Part model, mm, in its own coordinate system. Round coordinates to 2 decimals unless told otherwise and drop trailing zeros. Write each loop counter-clockwise with the first axis right and the second up, starting at its lowest first coordinate (ties: lowest second). Pieces come first, ordered by that corner, then holes. Notation, with made-up numbers: (82, -28) -> (91, -28) arc R16 ccw to (91, 2) -> close; hole circle Ø4 at (-9, 21). An arc over 180 degrees is marked (long way). Return JSON: item names as keys, results as strings. Group by question number.
(1) Drill centre lines: L1, parallel to Y at x = 18, z = 0.3; L2, parallel to Y at x = 15.25, z = 0.7; L3, parallel to X at y = -15, z = 1.25. Where is each one in solid material? Low to high. Write a range as from..to.
(2) Saw through at A-A (y = -15.25). List the corners of the cut face in (x, z), plus the area to 3 significant figures.
(3) Saw through at D-D (x = 5). List the corners of the cut face in (y, z).
(4) Saw through at B-B (x = -11). List the corners of the cut face in (y, z).
(5) Saw through at C-C (z = 0.8). State how many separate pieces and enclosed holes the cut face has, plus the area to 3 significant figures.
from build123d import *

# Parameters (mm, degrees)
F0_R     = 1.5
F0_R_2   = 3.25
F1_DEPTH = 1.5


# Not quite as in the source:
# - ends of sketch curves that miss each other by under 0.0002 mm in the source are joined


with BuildPart() as f1:
    # F0 (on Top) → F1 (new body)
    with BuildSketch(Plane.XY):
        with BuildLine():
            ThreePointArc((6.3250610024, 28.8463679906), (-4.837e-07, 28.033009), (-6.3250619384, 28.8463682354))
            Line((-6.3250619384, 28.8463682354), (-16.589434, 31.530609))
            ThreePointArc((-16.589434, 31.530609), (-20.910174001, 30.6508727545), (-22.854447, 26.693281))
            Line((-22.854447, 26.693281), (-22.854447, -26.693281))
            ThreePointArc((-22.854447, -26.693281), (-20.910174001, -30.6508727545), (-16.5894340018, -31.5306089933))
            Line((-16.5894340018, -31.5306089933), (-6.325062, -28.846368))
            ThreePointArc((-6.325062, -28.846368), (-4.837e-07, -28.033009), (6.3250610024, -28.8463679906))
            Line((6.3250610024, -28.8463679906), (16.589434, -31.530609))
            ThreePointArc((16.589434, -31.530609), (20.9101733838, -30.6508724589), (22.854446, -26.693281))
            Line((22.854446, -26.693281), (22.854446, 26.693281))
            ThreePointArc((22.854446, 26.693281), (20.9101733838, 30.6508724589), (16.5894339378, 31.530609238))
            Line((16.5894339378, 31.530609238), (6.3250610024, 28.8463679906))
        make_face()
        with Locations((-17.854447, -26.693281)):
            Circle(F0_R, mode=Mode.SUBTRACT)
        with Locations((-15.25, -15.25)):
            Circle(F0_R, mode=Mode.SUBTRACT)
        with Locations((-11, -3.5)):
            Circle(F0_R, mode=Mode.SUBTRACT)
        with Locations((5, -23.033009)):
            Circle(F0_R_2, mode=Mode.SUBTRACT)
        with Locations((17.854446, -26.693281)):
            Circle(F0_R, mode=Mode.SUBTRACT)
        with Locations((11, -3.5)):
            Circle(F0_R, mode=Mode.SUBTRACT)
        with Locations((15.25, -15.25)):
            Circle(F0_R, mode=Mode.SUBTRACT)
        with Locations((-15.25, 15.25)):
            Circle(F0_R, mode=Mode.SUBTRACT)
        with Locations((-11, 11.5)):
            Circle(F0_R, mode=Mode.SUBTRACT)
        with Locations((-17.854447, 26.693281)):
            Circle(F0_R, mode=Mode.SUBTRACT)
        with Locations((11, 11.5)):
            Circle(F0_R, mode=Mode.SUBTRACT)
        with Locations((15.25, 15.25)):
            Circle(F0_R, mode=Mode.SUBTRACT)
        with Locations((17.854446, 26.693281)):
            Circle(F0_R, mode=Mode.SUBTRACT)
    extrude(amount=F1_DEPTH)


solid = f1.part
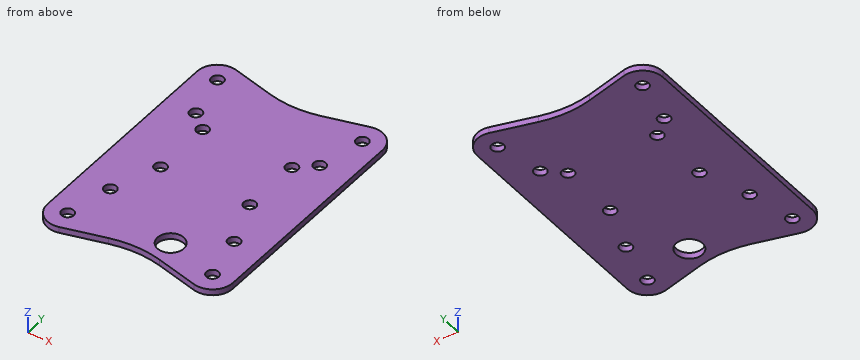
Computed values:
{
 "1": {"L1": "-31.69..-28.19, -25.2..25.2, 28.19..31.69", "L2": "-31.18..-16.75, -13.75..13.75, 16.75..31.18", "L3": "-22.85..-16.73, -13.77..13.77, 16.73..22.85"},
 "2": {"outline": "(-22.85, 0) -> (-16.75, 0) -> (-16.75, 1.5) -> (-22.85, 1.5) -> close; (-13.75, 0) -> (13.75, 0) -> (13.75, 1.5) -> (-13.75, 1.5) -> close; (16.75, 0) -> (22.85, 0) -> (22.85, 1.5) -> (16.75, 1.5) -> close", "area": "59.6 mm2"},
 "3": {"outline": "(-28.54, 0) -> (-26.28, 0) -> (-26.28, 1.5) -> (-28.54, 1.5) -> close; (-19.78, 0) -> (28.54, 0) -> (28.54, 1.5) -> (-19.78, 1.5) -> close"},
 "4": {"outline": "(-30.07, 0) -> (-5, 0) -> (-5, 1.5) -> (-30.07, 1.5) -> close; (-2, 0) -> (10, 0) -> (10, 1.5) -> (-2, 1.5) -> close; (13, 0) -> (30.07, 0) -> (30.07, 1.5) -> (13, 1.5) -> close"},
 "5": {"separate pieces": "1", "enclosed holes": "13", "area": "2,610 mm2"}
}
